Design review of the part built by this model. Coordinates are the model's own, in mm. Coordinates: 2 decimals unless noted, no trailing zeros. Loops run counter-clockwise (first coordinate to the right, second up) from the corner with the lowest first, then second, coordinate; pieces in that order, holes last. Notation, with made-up numbers: (52.5, -9.75) -> (96.5, -9.75) arc R21 cw to (96.5, 11.25) -> close; hole circle Ø6 at (76, 8). An arc over 180 degrees is marked (long way). Use one line per item in the form item = value. Start each with the question number.
1. Consider section A-A (y = 0). State the section outline as (x, z) points (3 decimals).
2. For pin 1 (6.5 mm diameter, centred on x = 127, y = -76.2, fed in from +Z); pin 2 (3 mm diameter, centred on y = -23, z = 3, fed in from -X); pin 3 (1.9 mm diameter, centred on y = -123.5, z = 3, fed in from +X); pin 4 (1.5 mm diameter, centred on y = -44, z = 0.5, fed in from -X), all flat-tipped, find the tip position at first contact; note any pin that passes through.
3. Consider section C-C (x = 35). State the section outline as (y, z) points, then the cut area to 3 significant figures.
4. Wall thickness on line 1 (Y direction, x = 57.15, z = 2.25); line 2 (X direction, y = 11, z = 6); line 3 (X direction, y = -43.5, z = 4): over which ranges is each line inside the solid? List them lowest first. Write a range as from..to.
5. Consider section D-D (x = 127). State how many separate pieces and enclosed holes the cut face has, then the cut area to 3 significant figures.
6. Consider section B-B (y = -82.55). State the section outline as (x, z) points, then the cut area to 3 significant figures.
from build123d import *

# Parameters (mm, degrees)
SKETCH1_R                          = 22.225
SKETCH1_R_2                        = 14.2875
SKETCH1_R_3                        = 12.065
BOSS_EXTRUDE1_DEPTH                = 6.35
F_9_0_196_DIAMETER_HOLE1_OUTLINE_R = 2.4892
F_9_0_196_DIAMETER_HOLE1_DEPTH     = 6.35
SKETCH5_W                          = 158.475738421
SKETCH5_H                          = 23.945509926
CUT_EXTRUDE1_DEPTH                 = 198.577920905
FILLET1_R                          = 12.7
SKETCH9_W                          = 50.8
SKETCH9_H                          = 25.4
CUT_EXTRUDE2_DEPTH                 = 198.577920905


# Read off the part's stored shape, not the designer's step: #9 (0.196) Diameter Hole1
with BuildPart() as part:
    # Sketch1 → Boss-Extrude1 (new body)
    with BuildSketch(Plane(origin=(0, 0, 0), x_dir=(0, 1, 0), z_dir=(0, 0, 1))):
        with BuildLine():
            Line((80.9625, -82.55), (80.9625, -139.7))
            Line((80.9625, -139.7), (-139.573, -139.7))
            Line((-139.573, -139.7), (-139.573, -8.2804))
            Line((-139.573, -8.2804), (-32.138994776, 54.766184957))
            ThreePointArc((-32.138994776, 54.766184957), (25.818013961, 58.014482288), (62.200093141, 12.782738878))
            Line((62.200093141, 12.782738878), (80.150058213, -74.560788201))
            ThreePointArc((80.150058213, -74.560788201), (80.758867143, -78.534792445), (80.9625, -82.55))
        make_face()
        with Locations(Location((0, 0, 0), (0, 0, 270))):
            Circle(SKETCH1_R, mode=Mode.SUBTRACT)
        with Locations(Location((-41.275, -82.55, 0), (0, 0, 270))):
            Circle(SKETCH1_R_2, mode=Mode.SUBTRACT)
        with Locations(Location((41.275, -82.55, 0), (0, 0, 270))):
            Circle(SKETCH1_R_2, mode=Mode.SUBTRACT)
        with Locations(Location((-82.55, -41.275, 0), (0, 0, 270))):
            Circle(SKETCH1_R_3, mode=Mode.SUBTRACT)
    extrude(amount=BOSS_EXTRUDE1_DEPTH)

    # #9 (0.196) Diameter Hole1 outline → #9 (0.196) Diameter Hole1 (cut)
    with BuildSketch(Plane.XY):
        with Locations((101.6, -127)):
            Circle(F_9_0_196_DIAMETER_HOLE1_OUTLINE_R)
        with Locations((114.3, -127)):
            Circle(F_9_0_196_DIAMETER_HOLE1_OUTLINE_R)
        with Locations((127, 63.5)):
            Circle(F_9_0_196_DIAMETER_HOLE1_OUTLINE_R)
        with Locations((127, 50.8)):
            Circle(F_9_0_196_DIAMETER_HOLE1_OUTLINE_R)
        with Locations((127, 38.1)):
            Circle(F_9_0_196_DIAMETER_HOLE1_OUTLINE_R)
        with Locations((127, 25.4)):
            Circle(F_9_0_196_DIAMETER_HOLE1_OUTLINE_R)
        with Locations((127, 12.7)):
            Circle(F_9_0_196_DIAMETER_HOLE1_OUTLINE_R)
        with Locations((127, 0)):
            Circle(F_9_0_196_DIAMETER_HOLE1_OUTLINE_R)
        with Locations((8.2804, -82.55)):
            Circle(F_9_0_196_DIAMETER_HOLE1_OUTLINE_R)
        with Locations((41.275, -121.031)):
            Circle(F_9_0_196_DIAMETER_HOLE1_OUTLINE_R)
        with Locations((74.2696, -82.55)):
            Circle(F_9_0_196_DIAMETER_HOLE1_OUTLINE_R)
        with Locations((0, -58.355558977)):
            Circle(F_9_0_196_DIAMETER_HOLE1_OUTLINE_R)
        with Locations((-10.779281546, -47.582226654)):
            Circle(F_9_0_196_DIAMETER_HOLE1_OUTLINE_R)
        with Locations((-17.965469244, -40.400005105)):
            Circle(F_9_0_196_DIAMETER_HOLE1_OUTLINE_R)
        with Locations((127, -12.7)):
            Circle(F_9_0_196_DIAMETER_HOLE1_OUTLINE_R)
        with Locations((127, -25.4)):
            Circle(F_9_0_196_DIAMETER_HOLE1_OUTLINE_R)
        with Locations((127, -38.1)):
            Circle(F_9_0_196_DIAMETER_HOLE1_OUTLINE_R)
        with Locations((127, -50.8)):
            Circle(F_9_0_196_DIAMETER_HOLE1_OUTLINE_R)
        with Locations((127, -63.5)):
            Circle(F_9_0_196_DIAMETER_HOLE1_OUTLINE_R)
        with Locations((127, -76.2)):
            Circle(F_9_0_196_DIAMETER_HOLE1_OUTLINE_R)
        with Locations((127, -88.9)):
            Circle(F_9_0_196_DIAMETER_HOLE1_OUTLINE_R)
        with Locations((127, -101.6)):
            Circle(F_9_0_196_DIAMETER_HOLE1_OUTLINE_R)
        with Locations((127, -114.3)):
            Circle(F_9_0_196_DIAMETER_HOLE1_OUTLINE_R)
        with Locations((127, -127)):
            Circle(F_9_0_196_DIAMETER_HOLE1_OUTLINE_R)
        with Locations((107.95, -41.275)):
            Circle(F_9_0_196_DIAMETER_HOLE1_OUTLINE_R)
        with Locations((82.55, -66.675)):
            Circle(F_9_0_196_DIAMETER_HOLE1_OUTLINE_R)
        with Locations((57.15, -41.275)):
            Circle(F_9_0_196_DIAMETER_HOLE1_OUTLINE_R)
        with Locations((82.55, -15.875)):
            Circle(F_9_0_196_DIAMETER_HOLE1_OUTLINE_R)
        with Locations((82.55, 15.875)):
            Circle(F_9_0_196_DIAMETER_HOLE1_OUTLINE_R)
        with Locations((107.95, 41.275)):
            Circle(F_9_0_196_DIAMETER_HOLE1_OUTLINE_R)
        with Locations((82.55, 66.675)):
            Circle(F_9_0_196_DIAMETER_HOLE1_OUTLINE_R)
        with Locations((57.15, 41.275)):
            Circle(F_9_0_196_DIAMETER_HOLE1_OUTLINE_R)
    extrude(amount=F_9_0_196_DIAMETER_HOLE1_DEPTH, mode=Mode.SUBTRACT)

    # Sketch5 → Cut-Extrude1 (cut, through all)
    with BuildSketch(Plane.XY.offset(6.35)):
        with Locations((102.364485766, 88.172754963)):
            Rectangle(SKETCH5_W, SKETCH5_H)
    extrude(amount=-CUT_EXTRUDE1_DEPTH, mode=Mode.SUBTRACT)

    # Fillet1
    fillet1_edges = [part.edges().sort_by_distance(p)[0] for p in [
        (8.2804, -139.573, 3.175),
        (55.340025647, 76.2, 3.175),
    ]]
    fillet(fillet1_edges, radius=FILLET1_R)

    # Sketch9 → Cut-Extrude2 (cut, through all)
    with BuildSketch(Plane.XY.offset(6.35)):
        with Locations((114.3, -126.873)):
            Rectangle(SKETCH9_W, SKETCH9_H)
    extrude(amount=-CUT_EXTRUDE2_DEPTH, mode=Mode.SUBTRACT)


solid = part.part
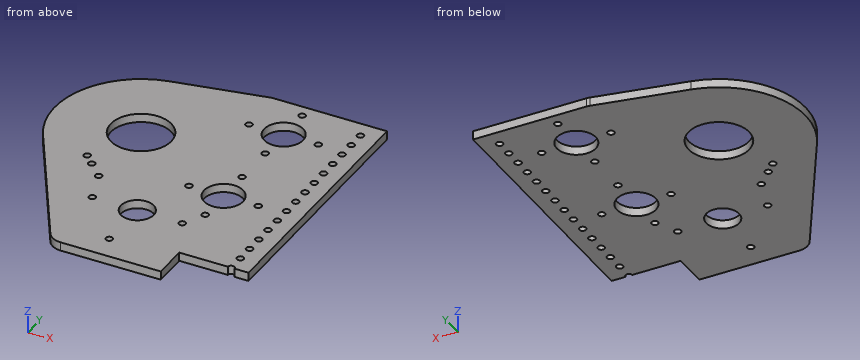
Geometry check:
q1.outline = (-63.5, 0) -> (-22.225, 0) -> (-22.225, 6.35) -> (-63.5, 6.35) -> close; (22.225, 0) -> (124.511, 0) -> (124.511, 6.35) -> (22.225, 6.35) -> close; (129.489, 0) -> (139.7, 0) -> (139.7, 6.35) -> (129.489, 6.35) -> close
q2.pin_1 = 6.35
q2.pin_2 = -59.75
q2.pin_3 = 88.9
q2.pin_4 = -48.25
q3.outline = (-139.57, 0) -> (-92.85, 0) -> (-92.85, 6.35) -> (-139.57, 6.35) -> close; (-72.25, 0) -> (72.02, 0) -> (72.02, 6.35) -> (-72.25, 6.35) -> close
q3.area = 1,210 mm²
q4.line_1 = -139.57..-43.76, -38.79..38.79, 43.76..76.2
q4.line_2 = -62.54..-19.31, 19.31..125.18, 128.82..139.7
q4.line_3 = -48.1..56.03, 58.27..68.44, 96.66..106.83, 109.07..139.7
q5.separate_pieces = 15
q5.enclosed_holes = 0
q5.area = 751 mm²
q6.outline = (-25.18, 0) -> (5.79, 0) -> (5.79, 6.35) -> (-25.18, 6.35) -> close; (10.77, 0) -> (29.21, 0) -> (29.21, 6.35) -> (10.77, 6.35) -> close; (53.34, 0) -> (71.78, 0) -> (71.78, 6.35) -> (53.34, 6.35) -> close; (76.76, 0) -> (139.7, 0) -> (139.7, 6.35) -> (76.76, 6.35) -> close
q6.area = 831 mm²
